from build123d import *

# Parameters (mm, degrees)
F0_W     = 2000
F0_H     = 500
F0_W_2   = 1860
F0_H_2   = 360
F1_DEPTH = 70
F2_W     = 30
F2_H     = 360
F3_DEPTH = 25
F4_DEPTH = 25
F5_W     = 360
F5_H     = 30
F6_DEPTH = 25


with BuildPart() as f1:
    # F0 (on Front) → F1 (new body)
    with BuildSketch(Plane.XZ):
        with Locations((18.946081, -353.424408)):
            Rectangle(F0_W, F0_H)
        with Locations((18.946081, -353.424408)):
            Rectangle(F0_W_2, F0_H_2, mode=Mode.SUBTRACT)
    extrude(amount=F1_DEPTH)



with BuildPart() as f3:
    # F2 (on face) → F3 (new body)
    with BuildSketch(Plane(origin=(0, 0, 0), x_dir=(-1, 0, 0), z_dir=(0, 1, 0))):
        with Locations((946.053919, -353.424408)):
            Rectangle(F2_W, F2_H)
    extrude(amount=-F3_DEPTH)


with BuildPart() as f1_1:
    add(f1.part)

    add(f3.part)  # F4 merges F3
    # F2 (on face) → F4 (join)
    with BuildSketch(Plane(origin=(0, 0, 0), x_dir=(-1, 0, 0), z_dir=(0, 1, 0))):
        with Locations((-983.946081, -353.424408)):
            Rectangle(F2_W, F2_H)
        with Locations((946.053919, -353.424408)):
            Rectangle(F2_W, F2_H)
    extrude(amount=F4_DEPTH)

    # F5 (on face) → F6 (cut)
    with BuildSketch(Plane.XY.offset(-103.424408)):
        with Locations((-601.053919, -35)):
            Rectangle(F5_W, F5_H)
    extrude(amount=-F6_DEPTH, mode=Mode.SUBTRACT)


solid = f1_1.part
The listing builds one solid part. Answer for the finished solid, in the listing's coordinates (mm). A direction names the side the tool comes from. Coordinates: 2 decimals unless noted, no trailing zeros. Order: outer loops, then holes, each group sorted by start corner. A loop starts at its lowest first (then second) coordinate and runs counter-clockwise, first axis right, second up. Notation, with made-up numbers: M -32.75,-17 L -15.75,-17 A24 cw -15.75,20 Z; hole C 15,-4.75 d5. An arc over 180 degrees is marked long. Use CSV: the item, a comma, the result in double quotes.
Q1. Section B-B (x = -39) is taken. Determine the outline of the cut face in (y, z).
Here are the results:
outline,"M -70,-603.42 L 0,-603.42 L 0,-533.42 L -70,-533.42 Z; M -70,-173.42 L 0,-173.42 L 0,-103.42 L -70,-103.42 Z"
Q2. Determine the mould class of faces 1 (the flat face through (1018.946, -35, -357)), 2 (the flat face through (5, -35, -603.424)), 3 (the flat face through (-911.054, -35, -356)) for opening direction Z: pulls with the +Z half, pulls with the -Z half, needs draft (parallel to the pull), parting line crosses it, or undercut.
Here are the results:
face 1,"needs draft"
face 2,"pulls with the -Z half"
face 3,"undercut"
Q3. A tool of negligible diameter and unlimited length cuts with its end or side. For faces 4 (the flat face through (6, -35, -173.424)), 5 (the flat face through (-981.054, -35, -357)), from which of +Z, -Z, +X, -X, +Y, -Y can it reach the whole face along a straight path? Write none if from no direction.
Here are the results:
face 4,"+Y, -Y"
face 5,"+Z, -Z, -X, +Y, -Y"
Q4. Given pin 1 Ø7.5 at (y, z) = (14.5, -434.5) entering from -X; pin 2 Ø12.5 at (x, y) = (979.5, 10) entering from +Z; pin 3 Ø20 at (x, z) = (-513, -116) entering from +Y, each flat-ended and moving along its own axis, determine where each tip first touches the part or whether it passes through.
Here are the results:
pin 1,"x = -961.05"
pin 2,"z = -173.42"
pin 3,"y = 0"
Q5. Straight lines are drawn through the part: L1, parallel to Z at x = -101, y = -19; L2, parallel to X at y = 5.5, z = -271.5; L3, parallel to X at y = -27, z = -492.5. For each, find the intervals that lie inside material, in ascending order.
Here are the results:
L1,"-603.42 to -533.42, -173.42 to -103.42"
L2,"-961.05 to -931.05, 968.95 to 998.95"
L3,"-981.05 to -911.05, 948.95 to 1018.95"
Q6. Section A-A (z = -266) is taken. Determine the outline of the cut face in (x, y).
Here are the results:
outline,"M -981.05,-70 L -911.05,-70 L -911.05,0 L -931.05,0 L -931.05,25 L -961.05,25 L -961.05,0 L -981.05,0 Z; M 948.95,-70 L 1018.95,-70 L 1018.95,0 L 998.95,0 L 998.95,25 L 968.95,25 L 968.95,0 L 948.95,0 Z"
Q7. Section C-C (y = -35.5) is taken. Determine the outline of the cut face in (x, z), then the cut area to 3 significant figures.
Here are the results:
outline,"M -981.05,-603.42 L 1018.95,-603.42 L 1018.95,-103.42 L -421.05,-103.42 L -421.05,-128.42 L -781.05,-128.42 L -781.05,-103.42 L -981.05,-103.42 Z; hole M -911.05,-533.42 L 948.95,-533.42 L 948.95,-173.42 L -911.05,-173.42 Z"
area,"321,000 mm2"
Q8. Section D-D (x = -655) is taken. Determine the outline of the cut face in (y, z).
Here are the results:
outline,"M -70,-603.42 L 0,-603.42 L 0,-533.42 L -70,-533.42 Z; M -70,-173.42 L 0,-173.42 L 0,-103.42 L -20,-103.42 L -20,-128.42 L -50,-128.42 L -50,-103.42 L -70,-103.42 Z"
